```python
from build123d import *

# Parameters (mm, degrees)
BLANKSKE_W          = 200
BLANKSKE_H          = 19
BLANK_DEPTH         = 20
TOOTHCUTSIM_DEPTH   = 202.893536301
TEETHCUTS_COUNT     = 43
TEETHCUTS_PITCH     = 4.712388975
SKETCH3_W           = 7
SKETCH3_H           = 7
BOSS_EXTRUDE2_DEPTH = 10
SKETCH4_W           = 3.3
SKETCH4_H           = 3.3
CUT_EXTRUDE1_DEPTH  = 25


with BuildPart() as part:
    # BlankSke → Blank (new body)
    with BuildSketch(Plane.XY):
        with Locations((100, 9.5)):
            Rectangle(BLANKSKE_W, BLANKSKE_H)
    extrude(amount=-BLANK_DEPTH)

    # TooCutSkeSim → ToothCutSim (cut, through all)
    with BuildSketch(Plane.XY):
        Polygon((0.654653055, 15.625), (-0.654653055, 15.625), (-1.892297439, 19.0254), (1.892297439, 19.0254), align=None)
    toothcutsim = extrude(amount=-TOOTHCUTSIM_DEPTH, mode=Mode.SUBTRACT)

    # TeethCuts: ToothCutSim ×43
    with Locations(*[(i * TEETHCUTS_PITCH, 0, 0) for i in range(1, TEETHCUTS_COUNT)]):
        add(toothcutsim, mode=Mode.SUBTRACT)

    # Sketch3 → Boss-Extrude2 (add)
    with BuildSketch(Plane.ZY):
        with Locations((-10, 7.8125)):
            Rectangle(SKETCH3_W, SKETCH3_H)
    extrude(amount=BOSS_EXTRUDE2_DEPTH)

    # Sketch4 → Cut-Extrude1 (cut)
    with BuildSketch(Plane(origin=(0, 0, -13.5), x_dir=(-1, 0, 0), z_dir=(0, 0, -1))):
        with Locations((5, 7.8125)):
            Rectangle(SKETCH4_W, SKETCH4_H)
    extrude(amount=-CUT_EXTRUDE1_DEPTH, mode=Mode.SUBTRACT)


solid = part.part
```
For this review, take the finished solid that the model builds, in its own axes (mm). A direction names the side the tool comes from. Give positions to 0.01 mm unless a question says otherwise; leave off trailing zeros. Answer as CSV lines item,"result".
1. For pin 1 (0.7 mm diameter, centred on x = 127.5, z = -14, fed in from +Y) (3 decimals); pin 2 (3 mm diameter, centred on y = 15.5, z = -12.5, fed in from -X), all flat-tipped, find the tip position at first contact; note any pin that passes through.
Findings:
pin 1,"stops at y = 15.625"
pin 2,"stops at x = 0"
2. Wall thickness on line 1 (X direction, y = 14.75, z = -5); line 2 (Y direction, x = 160, z = -1.5) (3 decimals): over which ranges is each line inside the solid? List them lowest first.
Findings:
line 1,"x = 0 to 200"
line 2,"y = 0 to 15.625"
3. Draft analysis for pull direction X (two halves, no side actions). For faces 1 (the flat face through (53.1, 17.3, -9.9)), 2 (the flat face through (1.28, 17.34, -9.86)), 3 (the flat face through (99, 10, 0)), 4 (the flat face through (121.26, 17.29, -9.86)), state which applies: +X half, -X half, draft (parallel to the pull), parting line (faces both ways), or undercut.
Findings:
face 1,"undercut"
face 2,"-X half"
face 3,"draft"
face 4,"undercut"
4. For faces 5 (the flat face through (-6.65, 8, -10)), 6 (the flat face through (109.662, 17.336, -9.86)), list the 3-axis set-ups (+Z, -Z, +X, -X, +Y, -Y) from which the entire face can be reached by the end or side of a thin tool; tool diameter is ignored.
Findings:
face 5,"+Z, -Z"
face 6,"+Z, -Z, +Y"
